Source: CAD feature listing. Evaluate the final solid. Frame: model axes, mm. A direction names the side the tool comes from. Round coordinates to 2 decimals unless told otherwise and drop trailing zeros. Write each loop counter-clockwise with the first axis right and the second up, starting at its lowest first coordinate (ties: lowest second). Pieces come first, ordered by that corner, then holes. Notation, with made-up numbers: M 21,-25.75 L 66,-25.75 A27 ccw 66,-1.75 Z; hole C 3,35 d10. An arc over 180 degrees is marked long. Answer in a Markdown table with one row per item. Add a question column.
Item 1: Cut plane B-B on x = 120.5. Return loops of the section in (y, z).
Item 2: Cut plane C-C on z = 30.5. Return loops of the section in (x, y).
Item 3: Contact query for flat-ended pins moving along their axis: pin 1 (6 mm diameter, centred on y = -12.5, z = 26, fed in from -X); pin 2 (8 mm diameter, centred on x = 104, y = -3.5, fed in from +Z); pin 3 (20 mm diameter, centred on y = -25.5, z = 21, fed in from +X). Output: stop coordinate, or through.
Item 4: Cut plane A-A on y = -17. Return loops of the section in (x, z), and give its area (3 significant figures).
Item 5: Set-up query: faces 1 (the face through (47, -20, 20)), 2 (the face through (168, 10, 11)), 3 (the face through (217.124, -2.465, 79.624)). Return all of +Z, -Z, +X, -X, +Y, -Y with unobstructed straight access to the full face (end or side cutting, diameter ignored); none if empty.
Item 6: Mould query, pull axis Z, two halves, no side actions, for faces 4 (the face through (201, -12.5, 68)), 5 (the face through (131.17, -19.72, 45.72)), 6 (the face through (1, -20, 18)). Classes: released by +Z, released by -Z, zero draft, split by the parting line, or undercut.
Item 7: Cut plane D-D on y = 13. Return loops of the section in (x, z).
Item 8: Material intervals for probe 1 along Y at (x, z) = (191, 31); probe 2 along Z at (x, y) = (37.5, -15.5); probe 3 along X at (y, z) = (-35, 31.5), sorted ascending.
from build123d import *

# Parameters (mm, degrees)
F1_DEPTH  = 40
F2_R      = 5
F7_DEPTH  = 5
F9_DEPTH  = 5
F10_W     = 40
F10_H     = 15
F11_DEPTH = 11.684
F3_R      = 2
F12_DEPTH = 20
F4_R      = 2
F13_DEPTH = 20


# Not quite as in the source:
# - two fillets or chamfers of one size are made in one step


with BuildPart() as f1:
    # F0 (on Front) → F1 (new body)
    with BuildSketch(Plane.XZ):
        with BuildLine():
            Line((0, 20), (0, 0))
            Line((0, 0), (200, 0))
            Line((200, 0), (200, 60))
            Line((200, 60), (180, 60))
            ThreePointArc((180, 60), (178.3255687097, 58.1433963871), (176.6122992708, 56.3225710381))
            ThreePointArc((176.6122992708, 56.3225710381), (138.7955155822, 29.9352120782), (93.7655988336, 20))
            ThreePointArc((93.7655988336, 20), (91.2655988336, 19.9735969417), (88.7655988336, 20))
            Line((88.7655988336, 20), (0, 20))
        make_face()
        with BuildLine():
            ThreePointArc((180, 60), (130.1910752068, 49.5607362037), (88.7655988336, 20))
            ThreePointArc((88.7655988336, 20), (91.2655988336, 19.9735969417), (93.7655988336, 20))
            ThreePointArc((93.7655988336, 20), (131.7599412204, 45.9823724222), (176.6122992708, 56.3225710381))
            ThreePointArc((176.6122992708, 56.3225710381), (178.3255687097, 58.1433963871), (180, 60))
        make_face()
        Polygon((180, 60), (200, 60), (229.4970817654, 81.2315874186), (222.6715144816, 90.714360058), align=None)
    extrude(amount=F1_DEPTH)

    # F2
    f2_edges = [f1.edges().sort_by_distance(p)[0] for p in [
        (0, -20, 20),
        (0, -20, 0),
        (200, -20, 0),
        (180, -20, 60),
    ]]
    fillet(f2_edges, radius=F2_R)

    # F6 (on face) → F7 (cut)
    with BuildSketch(Plane.XZ.offset(40)):
        Polygon((181.2943636671, 60.931664887), (200, 60), (220.5845981647, 74.8165062187), (213.7590308809, 84.2992788581), align=None)
    extrude(amount=-F7_DEPTH, mode=Mode.SUBTRACT)

    # F8 (on face) → F9 (cut)
    with BuildSketch(Plane(origin=(0, 0, 0), x_dir=(-1, 0, 0), z_dir=(0, 1, 0))):
        Polygon((-220.5845981647, 74.8165062187), (-200, 60), (-181.2943636671, 60.931664887), (-213.7590308809, 84.2992788581), align=None)
    extrude(amount=-F9_DEPTH, mode=Mode.SUBTRACT)

    # F10 (on face) → F11 (cut)
    with BuildSketch(Plane(origin=(32.9817876356, 0, -45.8216556055), x_dir=(0.8116166803, 0, 0.5841903493), z_dir=(-0.5841903493, 0, 0.8116166803))):
        with Locations((202.737220197, -20)):
            Rectangle(F10_W, F10_H)
    extrude(amount=-F11_DEPTH, mode=Mode.SUBTRACT)

    # F3 (on face) → F12 (join)
    with BuildSketch(Plane.XZ.offset(40)):
        with Locations((32, 11)):
            Circle(F3_R)
        with Locations((166, 11)):
            Circle(F3_R)
    extrude(amount=F12_DEPTH)

    # F4 (on face) → F13 (join)
    with BuildSketch(Plane(origin=(0, 0, 0), x_dir=(-1, 0, 0), z_dir=(0, 1, 0))):
        with Locations((-166, 11)):
            Circle(F4_R)
        with Locations((-34, 11)):
            Circle(F4_R)
    extrude(amount=F13_DEPTH)


solid = f1.part
Results below:
| question | item | result |
|---|---|---|
| 1 | outline | M -40,0 L 0,0 L 0,23.64 L -40,23.64 Z; M -40,40.35 L 0,40.35 L 0,44.8 L -40,44.8 Z |
| 2 | outline | M 99.7,-40 L 105.68,-40 L 105.68,0 L 99.7,0 Z; M 140.06,-40 L 200,-40 L 200,0 L 140.06,0 Z |
| 3 | pin 1 | x = 91.62 |
| 3 | pin 2 | z = 36.97 |
| 3 | pin 3 | x = 200 |
| 4 | outline | M 0,5 A5 ccw 5,0 L 195,0 A5 ccw 200,5 L 200,60 L 188.12,51.45 L 181.29,60.93 A5 cw 178.44,59.99 A124.05 ccw 88.77,20 L 5,20 A5 ccw 0,15 Z; M 213.76,84.3 L 220.58,74.82 L 229.5,81.23 L 222.67,90.71 Z; hole M 93.77,20 A118.37 ccw 176.61,56.32 A124.05 ccw Z |
| 4 | area | 6,300 mm2 |
| 5 | face 1 | +Z, -X, +Y, -Y |
| 5 | face 2 | +Y |
| 5 | face 3 | -Z, -X, +Y |
| 6 | face 4 | zero draft |
| 6 | face 5 | undercut |
| 6 | face 6 | released by +Z |
| 7 | outline | C 34,11 d4; C 166,11 d4 |
| 8 | probe 1 | -40 to 0 |
| 8 | probe 2 | 0 to 20 |
| 8 | probe 3 | 100.89 to 106.99, 142.22 to 200 |
